Job drawing, mm, ordinate dimensions from the low corner. One solid piece. A direction names the side the tool comes from. Coordinates: 2 decimals unless noted, no trailing zeros. Write each loop counter-clockwise with the first axis right and the second up, starting at its lowest first coordinate (ties: lowest second). Pieces come first, ordered by that corner, then holes.
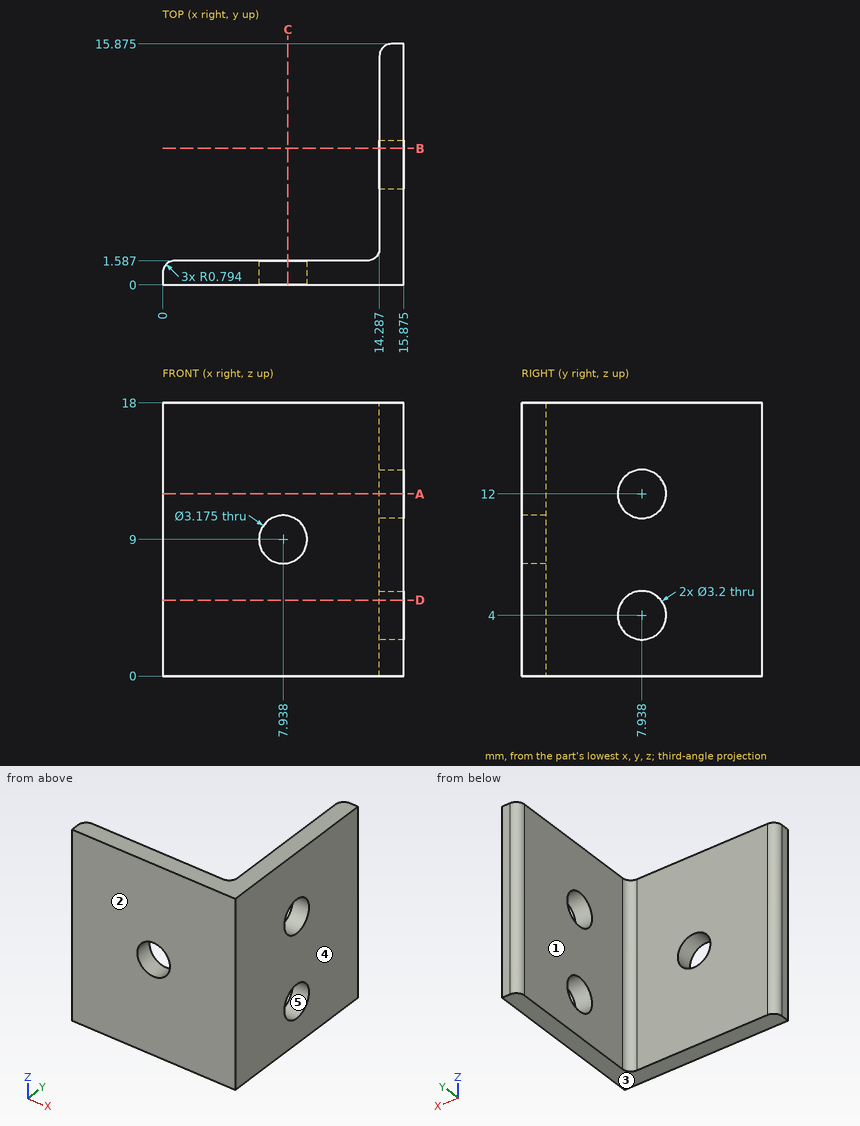
1. Saw through at C-C on x = 8.25. List the corners of the cut face in (y, z).
Computed values:
outline: (0, 0) - (1.59, 0) - (1.59, 7.44) - (0, 7.44) - close; (0, 10.56) - (1.59, 10.56) - (1.59, 18) - (0, 18) - close
2. Saw through at A-A on z = 12. List the corners of the cut face in (x, y) (1 decimal).
Computed values:
outline: (0, 0) - (15.9, 0) - (15.9, 6.3) - (14.3, 6.3) - (14.3, 2.4) arc R0.8 cw to (13.5, 1.6) - (0.8, 1.6) arc R0.8 ccw to (0, 0.8) - close; (14.3, 9.5) - (15.9, 9.5) - (15.9, 15.9) - (15.1, 15.9) arc R0.8 ccw to (14.3, 15.1) - close
3. Flat gauge pins, fed straight in: pin 1 (4 mm diameter, centred on x = 2, z = 2, fed in from +Y); pin 2 (8 mm diameter, centred on y = 6.5, z = 15, fed in from -X). Where does each tip first touch, or does it go through?
Computed values:
pin 1: stops at y = 1.59
pin 2: stops at x = 14.29
4. Saw through at B-B on y = 9. List the corners of the cut face in (x, z) (1 decimal).
Computed values:
outline: (14.3, 0) - (15.9, 0) - (15.9, 2.8) - (14.3, 2.8) - close; (14.3, 5.2) - (15.9, 5.2) - (15.9, 10.8) - (14.3, 10.8) - close; (14.3, 13.2) - (15.9, 13.2) - (15.9, 18) - (14.3, 18) - close
5. Saw through at D-D on z = 5. List the corners of the cut face in (x, y) (1 decimal).
Computed values:
outline: (0, 0) - (15.9, 0) - (15.9, 6.7) - (14.3, 6.7) - (14.3, 2.4) arc R0.8 cw to (13.5, 1.6) - (0.8, 1.6) arc R0.8 ccw to (0, 0.8) - close; (14.3, 9.2) - (15.9, 9.2) - (15.9, 15.9) - (15.1, 15.9) arc R0.8 ccw to (14.3, 15.1) - close
6. Probe line 1 along Y through (x, z) = (15.5, 4) (1 decimal); line 2 along Y through (x, z) = (1.25, 3); line 3 along X through (y, z) = (13.25, 6.75) (1 decimal). List the from-to ranges inside material, lowest first.
Computed values:
line 1: y = 0 to 6.3, 9.5 to 15.9
line 2: y = 0 to 1.59
line 3: x = 14.3 to 15.9
7. Mould opens along Z. For the marked faces 3, 4 and 5 say: +Z half, -Z half, draft (parallel to the pull), parting line (faces both ways), or undercut.
Computed values:
face 3: -Z half
face 4: draft
face 5: undercut
8. 3-axis set-ups, long thin cutter, end or side, ignore diameter. For the marked faces 1 and 2: which of +Z, -Z, +X, -X, +Y, -Y reach the whole face in a straight line?
Computed values:
face 1: +Z, -Z, -X, +Y
face 2: +Z, -Z, +X, -X, -Y
